```python
from build123d import *

# Parameters (mm, degrees)
ESQUISSE2_R             = 1.5
ENL_V_MAT_EXTRU_1_DEPTH = 10
CHANFREIN1_SIZE         = 1.5
ESQUISSE3_R             = 2
ENL_V_MAT_EXTRU_2_DEPTH = 10
CHANFREIN2_SIZE         = 0.2
CHANFREIN3_SIZE         = 0.5


with BuildPart() as part:
    # Esquisse1 → Révolution1 (revolve)
    with BuildSketch(Plane.XY, mode=Mode.PRIVATE) as r_volution1_sk:
        Polygon((-15, 0), (-25.5, 0), (-25.5, 8), (-19, 8), (-19, 40), (-9, 40), (-9, 36), (-15, 36), align=None)
    revolve(r_volution1_sk.sketch.rotate(Axis((0, 0, 0), (0, 1, 0)), 270), axis=Axis((0, 0, 0), (0, 1, 0)))

    # Esquisse2 → Enlèv. mat.-Extru.1 (cut)
    with BuildSketch(Plane(origin=(0, 40, 0), x_dir=(1, 0, 0), z_dir=(0, 1, 0))):
        with Locations(Location((-8.75, 8.75, 0), (0, 0, 270))):
            Circle(ESQUISSE2_R)
        with Locations(Location((8.75, 8.75, 0), (0, 0, 270))):
            Circle(ESQUISSE2_R)
        with Locations(Location((8.75, -8.75, 0), (0, 0, 270))):
            Circle(ESQUISSE2_R)
        with Locations(Location((-8.75, -8.75, 0), (0, 0, 270))):
            Circle(ESQUISSE2_R)
    extrude(amount=-ENL_V_MAT_EXTRU_1_DEPTH, mode=Mode.SUBTRACT)

    # Chanfrein1
    chanfrein1_edges = [part.edges().sort_by_distance(p)[0] for p in [
        (-8.75, 40, -10.25),
        (8.75, 40, -10.25),
        (8.75, 40, 7.25),
        (-8.75, 40, 7.25),
    ]]
    chamfer(chanfrein1_edges, length=CHANFREIN1_SIZE)

    # Esquisse3 → Enlèv. mat.-Extru.2 (cut)
    with BuildSketch(Plane(origin=(0, 8, 0), x_dir=(1, 0, 0), z_dir=(0, 1, 0))):
        with Locations(Location((-22.5, 0, 0), (0, 0, 270))):
            Circle(ESQUISSE3_R)
        with Locations(Location((22.5, 0, 0), (0, 0, 270))):
            Circle(ESQUISSE3_R)
    extrude(amount=-ENL_V_MAT_EXTRU_2_DEPTH, mode=Mode.SUBTRACT)

    # Chanfrein2
    chanfrein2_edges = [part.edges().sort_by_distance(p)[0] for p in [
        (-8.75, 36, -10.25),
        (8.75, 36, -10.25),
        (8.75, 36, 7.25),
        (-8.75, 36, 7.25),
        (-22.5, 0, -2),
        (-22.5, 8, -2),
        (22.5, 0, -2),
        (22.5, 8, -2),
    ]]
    chamfer(chanfrein2_edges, length=CHANFREIN2_SIZE)

    # Chanfrein3
    # the kernel refuses this chamfer: 0.5 mm, written as the material it adds along each edge
    with BuildSketch(Plane(origin=(0, 36, 0), x_dir=(0, 0, -1), z_dir=(1, 0, 0))) as chanfrein3_piece_1:
        Polygon((15 - CHANFREIN3_SIZE, 0), (15, -CHANFREIN3_SIZE), (15, 0), align=None)
    revolve(axis=Axis((0, 36, 0), (0, 1, 0)))
    with BuildSketch(Plane(origin=(0, 8, 0), x_dir=(0, 0, -1), z_dir=(1, 0, 0))) as chanfrein3_piece_2:
        Polygon((19, CHANFREIN3_SIZE), (19 + CHANFREIN3_SIZE, 0), (19, 0), align=None)
    revolve(axis=Axis((0, 8, 0), (0, 1, 0)))
    # the kernel refuses this chamfer: 0.5 mm, written as the material it takes off along each edge
    with BuildSketch(Plane(origin=(0, 36, 0), x_dir=(0, 0, -1), z_dir=(1, 0, 0))) as chanfrein3_2_piece_1:
        Polygon((9 + CHANFREIN3_SIZE, 0), (9, CHANFREIN3_SIZE), (9, 0), align=None)
    revolve(axis=Axis((0, 36, 0), (0, 1, 0)), mode=Mode.SUBTRACT)
    with BuildSketch(Plane(origin=(0, 40, 0), x_dir=(0, 0, -1), z_dir=(1, 0, 0))) as chanfrein3_2_piece_2:
        Polygon((9 + CHANFREIN3_SIZE, 0), (9, -CHANFREIN3_SIZE), (9, 0), align=None)
    revolve(axis=Axis((0, 40, 0), (0, 1, 0)), mode=Mode.SUBTRACT)
    with BuildSketch(Plane(origin=(0, 40, 0), x_dir=(0, 0, -1), z_dir=(1, 0, 0))) as chanfrein3_2_piece_3:
        Polygon((19 - CHANFREIN3_SIZE, 0), (19, -CHANFREIN3_SIZE), (19, 0), align=None)
    revolve(axis=Axis((0, 40, 0), (0, 1, 0)), mode=Mode.SUBTRACT)
    with BuildSketch(Plane(origin=(0, 8, 0), x_dir=(0, 0, -1), z_dir=(1, 0, 0))) as chanfrein3_2_piece_4:
        Polygon((25.5 - CHANFREIN3_SIZE, 0), (25.5, -CHANFREIN3_SIZE), (25.5, 0), align=None)
    revolve(axis=Axis((0, 8, 0), (0, 1, 0)), mode=Mode.SUBTRACT)
    with BuildSketch(Plane(origin=(0, 0, 0), x_dir=(0, 0, -1), z_dir=(1, 0, 0))) as chanfrein3_2_piece_5:
        Polygon((25.5 - CHANFREIN3_SIZE, 0), (25.5, CHANFREIN3_SIZE), (25.5, 0), align=None)
    revolve(axis=Axis((0, 0, 0), (0, 1, 0)), mode=Mode.SUBTRACT)
    with BuildSketch(Plane(origin=(0, 0, 0), x_dir=(0, 0, -1), z_dir=(1, 0, 0))) as chanfrein3_2_piece_6:
        Polygon((15, CHANFREIN3_SIZE), (15 + CHANFREIN3_SIZE, 0), (15, 0), align=None)
    revolve(axis=Axis((0, 0, 0), (0, 1, 0)), mode=Mode.SUBTRACT)


solid = part.part
```
CAD build for the part. Positions are in the model's coordinates, mm. A direction names the side the tool comes from. Round coordinates to 2 decimals unless told otherwise and drop trailing zeros. Write each loop counter-clockwise with the first axis right and the second up, starting at its lowest first coordinate (ties: lowest second). Pieces come first, ordered by that corner, then holes.
Item 1: Band-saw the part on B-B on y = 24. Write the cut outline in (x, z).
Filled in:
outline: circle Ø38 at (0, 0); hole circle Ø30 at (0, 0)
Item 2: Drill centre lines: L1, parallel to X at y = 3, z = 0; L2, parallel to X at y = 37, z = 0; L3, parallel to Y at x = -15.5, z = 19. Where is each one in solid material? Low to high.
Filled in:
L1: x = -25.5 to -24.5, -20.5 to -15, 15 to 20.5, 24.5 to 25.5
L2: x = -19 to -9, 9 to 19
L3: y = 0 to 8
Item 3: Tool access for faces 3 (the flat face through (9.5, 36, 3)), 4 (the flat face through (12, 40, 0)): list every direction of +Z, -Z, +X, -X, +Y, -Y with a clear straight run to the whole face (end or side of a thin tool).
Filled in:
face 3: -Y
face 4: +Z, -Z, +X, -X, +Y
Item 4: Mould opens along X. For faces 1 (the cylindrical face through (-9.66, 37.37, -9.94)), 2 (the flat face through (-11.5, 0, 10.8)) say: released by +X, released by -X, zero draft, split by the parting line, or undercut.
Filled in:
face 1: undercut
face 2: zero draft
Item 5: Band-saw the part on D-D on y = 4. Write the cut outline in (x, z), then the cut area to 3 significant figures.
Filled in:
outline: circle Ø51 at (0, 0); hole circle Ø4 at (-22.5, 0); hole circle Ø30 at (0, 0); hole circle Ø4 at (22.5, 0)
area: 1,310 mm2
Item 6: Band-saw the part on C-C on z = 0. Give the number of separate pieces and of enclosed holes in the cut face, then the cut area to 3 significant figures.
Filled in:
separate pieces: 4
enclosed holes: 0
area: 407 mm2
Item 7: Drop flat-ended pins along their axis: pin 1 Ø8.5 at (x, z) = (-5, -0.5) entering from -Y; pin 2 Ø5 at (x, z) = (8.75, -8.75) entering from -Y; pin 3 Ø5 at (x, y) = (14.5, 33) entering from -Z. Give the stop position or say it passes through.
Filled in:
pin 1: stops at y = 36.23
pin 2: stops at y = 35.63
pin 3: stops at z = -14.73
